Check sheet for the modelled part. Datum: model origin and axes. Units: mm. Face numbers are marked on the shaded views. A direction names the side the tool comes from. Give positions to 0.01 mm unless a question says otherwise; leave off trailing zeros. Order: outer loops, then holes, each group sorted by start corner. A loop starts at its lowest first (then second) coordinate and runs counter-clockwise, first axis right, second up.
```python
from build123d import *
from build123d.topology import SkipClean

# Parameters (mm, degrees)
SKETCH1_R           = 15.75
BOSS_EXTRUDE1_DEPTH = 10
CUT_EXTRUDE1_DEPTH  = 10
BOSS_EXTRUDE2_START = 3
BOSS_EXTRUDE2_DEPTH = 3
CHAMFER1_SIZE       = 0.2


with BuildPart() as part:
    # Sketch1 → Boss-Extrude1 (new body)
    with BuildSketch(Plane(origin=(0, 0, 0), x_dir=(1, 0, 0), z_dir=(0, 1, 0))):
        with Locations(Location((0, 0, 0), (0, 0, 270))):
            Circle(SKETCH1_R)
    extrude(amount=BOSS_EXTRUDE1_DEPTH)

    # Sketch2 → Cut-Extrude1 (cut)
    with BuildSketch(Plane(origin=(0, 10, 0), x_dir=(1, 0, 0), z_dir=(0, 1, 0))):
        Polygon((3.274663124, 3.655121716), (-1.528096697, 4.663502312), (-4.802759822, 1.008380597), (-3.274663124, -3.655121716), (1.528096697, -4.663502312), (4.802759822, -1.008380597), align=None)
    extrude(amount=-CUT_EXTRUDE1_DEPTH, mode=Mode.SUBTRACT)

    # Sketch3 → Boss-Extrude2 (add)
    with SkipClean():  # the faces are left unmerged after this step: merging them gives an invalid solid
        with BuildSketch(Plane.XZ.offset(BOSS_EXTRUDE2_START)):
            with BuildLine():
                Line((-11.155612536, -11.118219684), (-7.154915715, -3.105991164))
                Line((-7.154915715, -3.105991164), (-15.740134193, -0.557382799))
                ThreePointArc((-15.740134193, -0.557382799), (-14.447425963, -6.271712927), (-11.155612536, -11.118219684))
            make_face()
            with BuildLine():
                Line((-0.887590606, -7.749334353), (-7.387359433, -13.910047469))
                ThreePointArc((-7.387359433, -13.910047469), (-1.792250262, -15.647694367), (4.050854423, -15.220153693))
                Line((4.050854423, -15.220153693), (-0.887590606, -7.749334353))
            make_face()
            with BuildLine():
                Line((6.267325109, -4.643343189), (8.35277476, -13.352664671))
                ThreePointArc((8.35277476, -13.352664671), (12.655175702, -9.37598144), (15.206466959, -4.101934009))
                Line((15.206466959, -4.101934009), (6.267325109, -4.643343189))
            make_face()
            with BuildLine():
                ThreePointArc((15.740134193, 0.557382799), (14.447425963, 6.271712927), (11.155612536, 11.118219684))
                Line((11.155612536, 11.118219684), (7.154915715, 3.105991164))
                Line((7.154915715, 3.105991164), (15.740134193, 0.557382799))
            make_face()
            with BuildLine():
                ThreePointArc((7.387359433, 13.910047469), (1.792250262, 15.647694367), (-4.050854423, 15.220153693))
                Line((-4.050854423, 15.220153693), (0.887590606, 7.749334353))
                Line((0.887590606, 7.749334353), (7.387359433, 13.910047469))
            make_face()
            with BuildLine():
                ThreePointArc((-8.35277476, 13.352664671), (-12.655175702, 9.37598144), (-15.206466959, 4.101934009))
                Line((-15.206466959, 4.101934009), (-6.267325109, 4.643343189))
                Line((-6.267325109, 4.643343189), (-8.35277476, 13.352664671))
            make_face()
        extrude(amount=-BOSS_EXTRUDE2_DEPTH)

    # Chamfer1
    chamfer1_edges = [part.edges().sort_by_distance(p)[0] for p in [
        (4.038711473, 10, -1.323370559),
        (0.873283214, 10, -4.159312014),
        (-3.16542826, 10, -2.835941455),
        (-4.038711473, 10, 1.323370559),
        (-0.873283214, 10, 4.159312014),
        (3.16542826, 10, 2.835941455),
        (-9.155264126, -3, -7.112105424),
        (-11.447524954, -3, -1.831686981),
        (1.581631909, -3, -11.484744023),
        (-4.13747502, -3, -10.829690911),
        (10.736896034, -3, -4.372638599),
        (7.310049935, -3, -8.99800393),
        (9.155264126, -3, 7.112105424),
        (11.447524954, -3, 1.831686981),
        (-1.581631909, -3, 11.484744023),
        (4.13747502, -3, 10.829690911),
        (-10.736896034, -3, 4.372638599),
        (-7.310049935, -3, 8.99800393),
    ]]
    chamfer(chamfer1_edges, length=CHAMFER1_SIZE)


solid = part.part
```
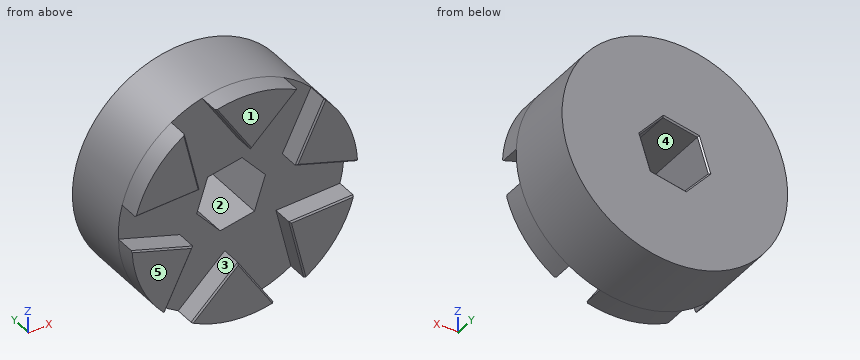
(1) Cross-section at A-A on y = -0.75. Enter the section's corners in (x, z).
Response values:
outline: (-15.74, -0.56) arc R15.75 ccw to (-11.16, -11.12) - (-7.15, -3.11) - close; (-15.21, 4.1) - (-6.27, 4.64) - (-8.35, 13.35) arc R15.75 ccw to start; (-7.39, -13.91) arc R15.75 ccw to (4.05, -15.22) - (-0.89, -7.75) - close; (-4.05, 15.22) - (0.89, 7.75) - (7.39, 13.91) arc R15.75 ccw to start; (6.27, -4.64) - (8.35, -13.35) arc R15.75 ccw to (15.21, -4.1) - close; (7.15, 3.11) - (15.74, 0.56) arc R15.75 ccw to (11.16, 11.12) - close
(2) Cross-section at C-C on y = 6.75. Enter the section's corners in (x, z), then the cut area to 3 significant figures.
Response values:
outline: circle Ø31.5 at (0, 0); hole (-4.8, -1.01) - (-1.53, -4.66) - (3.27, -3.66) - (4.8, 1.01) - (1.53, 4.66) - (-3.27, 3.66) - close
area: 717 mm2
(3) Release check for a two-part mould opening along Z. For the marked faces 4 and 5 record: released by +Z, released by -Z, zero draft, split by the parting line, or undercut.
Response values:
face 4: undercut
face 5: zero draft
(4) Set-up check for the marked faces 1, 2 and 3: record each of +Z, -Z, +X, -X, +Y, -Y from which the full face is reachable in a straight line by a thin tool's end or side.
Response values:
face 1: +Z, -Z, +X, -X, -Y
face 2: +Y, -Y
face 3: -Y
(5) Cross-section at B-B on z = 0. Enter the section's corners in (x, y).
Response values:
outline: (-15.75, 0) - (-4.47, 0) - (-4.47, 9.8) - (-4.68, 10) - (-15.75, 10) - close; (4.47, 0) - (15.75, 0) - (15.75, 10) - (4.68, 10) - (4.47, 9.8) - close
(6) Gauge pin test, flat ends, axial feed: pin 1 Ø1.5 at (y, z) = (8.5, 5) entering from -X; pin 2 Ø3 at (x, y) = (-10, 7) entering from -Z; pin 3 Ø1.5 at (y, z) = (4, -8) entering from -X. Record the tip position at first contact, or that the pin passes through.
Response values:
pin 1: stops at x = -15.17
pin 2: stops at z = -13.26
pin 3: stops at x = -13.98
(7) Material ranges on L1, parallel to Y at x = -7.5, z = -4; L2, parallel to X at y = 9.5, z = 2; L3, parallel to Z at x = 10, y = -1.5, recorded low to high.
Response values:
L1: y = 0 to 10
L2: x = -15.62 to -3.82, 3.91 to 15.62
L3: z = -12.17 to -4.42, 2.26 to 8.8
(8) Cross-section at D-D on x = 0. Enter the section's corners in (y, z), then the cut area to 3 significant figures.
Response values:
outline: (-3, -15.75) - (10, -15.75) - (10, -4.55) - (9.8, -4.34) - (0, -4.34) - (0, -9.09) - (-2.8, -9.09) - (-3, -9.45) - close; (-3, 9.45) - (-2.8, 9.09) - (0, 9.09) - (0, 4.34) - (9.8, 4.34) - (10, 4.55) - (10, 15.75) - (-3, 15.75) - close
area: 268 mm2
